Design review of the part built by this model. Coordinates are the model's own, in mm. Face numbers are marked on the shaded views. A direction names the side the tool comes from. Give positions to 0.01 mm unless a question says otherwise; leave off trailing zeros. Loops run counter-clockwise (first coordinate to the right, second up) from the corner with the lowest first, then second, coordinate; pieces in that order, holes last. Notation, with made-up numbers: (67, -16.75) -> (107, -16.75) arc R19 cw to (107, 15.25) -> close; hole circle Ø8 at (24.5, -28). An arc over 180 degrees is marked (long way). Use a Markdown table: item, result. Add a question column.
1. Add section C-C (z = -3.5). State the section outline as (x, y) points, and give its area (3 significant figures).
2. Add section A-A (x = 0). State the section outline as (y, z) points.
3. For pin 1 Ø6 at (y, z) = (3, 3.5) entering from +X; pin 2 Ø5 at (x, y) = (-4.5, 4.5) entering from +Z; pin 3 Ø1.5 at (x, y) = (0, 13) entering from +Z, all flat-tipped, find the tip position at first contact; note any pin that passes through.
4. For the marked faces 1, 2, 3, 4 and 5, list the 3-axis set-ups (+Z, -Z, +X, -X, +Y, -Y) from which the entire face can be reached by the end or side of a thin tool; tool diameter is ignored.
5. To check wall thickness, follow line 1 (Z direction, x = -0.25, y = 3.5); line 2 (Y direction, x = 0.75, z = 4); line 3 (Y direction, x = 1.75, z = 4). State the ranges of each line that lie inside material, in increasing order.
6. Draft analysis for pull direction Z (two halves, no side actions). For the marked faces 6, 7, 8 and 9, state which applies: pulls with the +Z half, pulls with the -Z half, needs draft (parallel to the pull), parting line crosses it, or undercut.
7. Add section B-B (y = 3.75). State the section outline as (x, z) points.
8. Add section D-D (z = 4). State the section outline as (x, y) points.
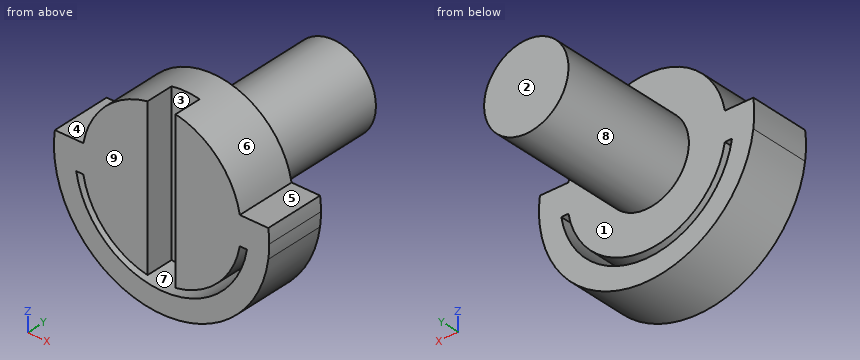
```python
from build123d import *

# Parameters (mm, degrees)
BOSS_EXTRUDE1_DEPTH = 4.3
SKETCH2_R           = 3
BOSS_EXTRUDE2_DEPTH = 10
SKETCH3_W           = 2
SKETCH3_H           = 11.870992598
CUT_EXTRUDE1_DEPTH  = 2


with BuildPart() as part:
    # Sketch1 → Boss-Extrude1 (new body)
    with BuildSketch(Plane(origin=(0, 0, 0), x_dir=(1, 0, 0), z_dir=(0, 1, 0))):
        with BuildLine():
            Line((5.560800302, -1), (-5.560800302, -1))
            ThreePointArc((-5.560800302, -1), (0, -5.65), (5.560800302, -1))
        make_face()
        with BuildLine():
            Line((5.560800302, 1), (-5.560800302, 1))
            ThreePointArc((-5.560800302, 1), (-5.65, 0), (-5.560800302, -1))
            Line((-5.560800302, -1), (5.560800302, -1))
            ThreePointArc((5.560800302, -1), (5.627655893, -0.501985205), (5.65, 0))
            ThreePointArc((5.65, 0), (5.627655893, 0.501985205), (5.560800302, 1))
        make_face()
        with BuildLine():
            ThreePointArc((5.560800302, 1), (0, 5.65), (-5.560800302, 1))
            Line((-5.560800302, 1), (5.560800302, 1))
        make_face()
        with BuildLine():
            Line((-5.560800302, 1), (-6.068154579, 1))
            ThreePointArc((-6.068154579, 1), (-6.15, 0), (-6.068154579, -1))
            Line((-6.068154579, -1), (-5.560800302, -1))
            ThreePointArc((-5.560800302, -1), (-5.65, 0), (-5.560800302, 1))
        make_face()
        with BuildLine():
            ThreePointArc((6.15, 0), (6.129504493, 0.501671873), (6.068154579, 1))
            Line((6.068154579, 1), (5.560800302, 1))
            ThreePointArc((5.560800302, 1), (5.627655893, 0.501985205), (5.65, 0))
            ThreePointArc((5.65, 0), (5.627655893, -0.501985205), (5.560800302, -1))
            Line((5.560800302, -1), (6.068154579, -1))
            ThreePointArc((6.068154579, -1), (6.129504493, -0.501671873), (6.15, 0))
        make_face()
        with BuildLine():
            Line((-6.068154579, 1), (-7.584358905, 1))
            ThreePointArc((-7.584358905, 1), (-7.65, 0), (-7.584358905, -1))
            Line((-7.584358905, -1), (-6.068154579, -1))
            ThreePointArc((-6.068154579, -1), (-6.15, 0), (-6.068154579, 1))
        make_face()
        with BuildLine():
            ThreePointArc((7.65, 0), (7.633572087, 0.50107603), (7.584358905, 1))
            Line((7.584358905, 1), (6.068154579, 1))
            ThreePointArc((6.068154579, 1), (6.129504493, 0.501671873), (6.15, 0))
            ThreePointArc((6.15, 0), (6.129504493, -0.501671873), (6.068154579, -1))
            Line((6.068154579, -1), (7.584358905, -1))
            ThreePointArc((7.584358905, -1), (7.633572087, -0.50107603), (7.65, 0))
        make_face()
        with BuildLine():
            ThreePointArc((7.584358905, 1), (0, 7.65), (-7.584358905, 1))
            Line((-7.584358905, 1), (-6.068154579, 1))
            ThreePointArc((-6.068154579, 1), (0, 6.15), (6.068154579, 1))
            Line((6.068154579, 1), (7.584358905, 1))
        make_face()
    extrude(amount=BOSS_EXTRUDE1_DEPTH)

    # Sketch2 → Boss-Extrude2 (add)
    with BuildSketch(Plane(origin=(0, 4.3, 0), x_dir=(1, 0, 0), z_dir=(0, 1, 0))):
        Circle(SKETCH2_R)
    extrude(amount=BOSS_EXTRUDE2_DEPTH)

    # Sketch3 → Cut-Extrude1 (cut)
    with BuildSketch(Plane.XZ):
        Rectangle(SKETCH3_W, SKETCH3_H)
    extrude(amount=-CUT_EXTRUDE1_DEPTH, mode=Mode.SUBTRACT)


solid = part.part
```
Taken from the geometry:
| question | item | result |
|---|---|---|
| 1 | outline | (-6.8, 0) -> (-5.06, 0) -> (-5.06, 4.3) -> (-6.8, 4.3) -> close; (-4.44, 0) -> (-1, 0) -> (-1, 2) -> (1, 2) -> (1, 0) -> (4.44, 0) -> (4.44, 4.3) -> (-4.44, 4.3) -> close; (5.06, 0) -> (6.8, 0) -> (6.8, 4.3) -> (5.06, 4.3) -> close |
| 1 | area | 49.2 mm^2 |
| 2 | outline | (0, -7.65) -> (4.3, -7.65) -> (4.3, -6.15) -> (0, -6.15) -> close; (2, -5.65) -> (4.3, -5.65) -> (4.3, -3) -> (14.3, -3) -> (14.3, 3) -> (4.3, 3) -> (4.3, 5.65) -> (2, 5.65) -> close |
| 3 | pin 1 | stops at x = 7.63 |
| 3 | pin 2 | stops at z = 5.28 |
| 3 | pin 3 | stops at z = 3 |
| 4 | face 1 | +Y |
| 4 | face 2 | +Z, -Z, +X, -X, +Y |
| 4 | face 3 | +Z, -Y |
| 4 | face 4 | +Z, -X, +Y, -Y |
| 4 | face 5 | +Z, +X, +Y, -Y |
| 5 | line 1 | z = -7.65 to -6.14, -5.64 to 5.64 |
| 5 | line 2 | y = 2 to 4.3 |
| 5 | line 3 | y = 0 to 4.3 |
| 6 | face 6 | pulls with the +Z half |
| 6 | face 7 | undercut |
| 6 | face 8 | parting line crosses it |
| 6 | face 9 | needs draft |
| 7 | outline | (-7.58, 1) arc R7.65 ccw (long way) to (7.58, 1) -> (5.56, 1) arc R5.65 ccw to (-5.56, 1) -> close; hole (-6.07, -1) arc R6.15 ccw to (6.07, -1) -> (5.56, -1) arc R5.65 cw to (-5.56, -1) -> close |
| 8 | outline | (-3.99, 0) -> (-1, 0) -> (-1, 2) -> (1, 2) -> (1, 0) -> (3.99, 0) -> (3.99, 4.3) -> (-3.99, 4.3) -> close |
